CAD build for the part. Positions are in the model's coordinates, mm. Face numbers are marked on the shaded views. Round coordinates to 2 decimals unless told otherwise and drop trailing zeros. Write each loop counter-clockwise with the first axis right and the second up, starting at its lowest first coordinate (ties: lowest second). Pieces come first, ordered by that corner, then holes. Notation, with made-up numbers: (38.5, 12.25) - (72.5, 12.25) arc R26 ccw to (72.5, 35.25) - close; hole circle Ø4 at (-10.5, 45). An arc over 180 degrees is marked (long way). Put each result on its own line as item: value. Start each with the question number.
Item 1: Cut at B-B (y = 20). Give the cut face in (x, z).
Item 2: Drill centre lines: line 1 (Y direction, x = -27.5, z = 2.75); line 2 (X direction, y = -9, z = 1.65); line 3 (Y direction, x = -4, z = 1.15). Where is each one in solid material? Low to high. Write a range as from..to.
Item 3: Cut at C-C (x = -50.5). Give the cut face in (y, z), and give its area (3 significant figures).
Item 4: Cut at A-A (z = 1.55). Count the separate pieces of the cut face and the enclosed holes in it, and give its area (3 significant figures).
Item 5: Pin check, flat tip, straight feed: pin 1 Ø1.5 at (y, z) = (10.5, 1.5) entering from +X. Stop position of the tip, or through.
Item 6: Mould opens along Z. For the marked faces 1 and 2 say: released by +Z, released by -Z, zero draft, split by the parting line, or undercut.
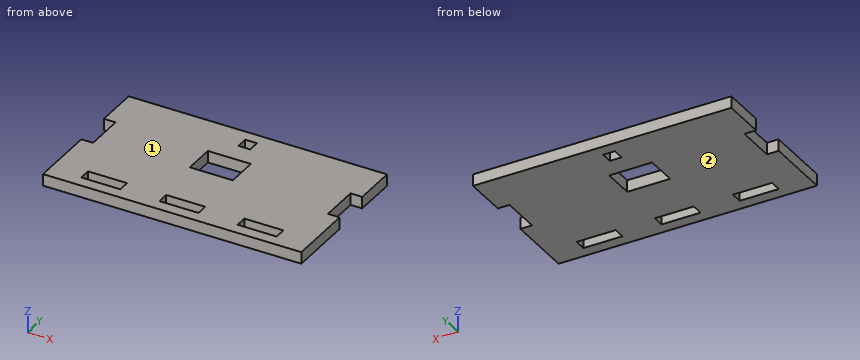
```python
from build123d import *

# Parameters (mm, degrees)
SKETCH1_W           = 10
SKETCH1_H           = 3
SKETCH1_W_2         = 11
SKETCH1_H_2         = 8
SKETCH1_W_3         = 3
BOSS_EXTRUDE1_DEPTH = 3


with BuildPart() as part:
    # Sketch1 → Boss-Extrude1 (new body)
    with BuildSketch(Plane.XY):
        Polygon((4.993890114, 24.809336695), (-61.106109886, 24.809336695), (-61.106109886, 13.809336695), (-58.106109886, 13.809336695), (-58.106109886, 3.809336695), (-61.106109886, 3.809336695), (-61.106109886, -13.190663305), (4.993890114, -13.190663305), (4.993890114, 3.809336695), (1.993890114, 3.809336695), (1.993890114, 13.809336695), (4.993890114, 13.809336695), align=None)
        with Locations((-28.056109886, -8.690663305)):
            Rectangle(SKETCH1_W, SKETCH1_H, mode=Mode.SUBTRACT)
        with Locations((-28.856109886, 9.559336695)):
            Rectangle(SKETCH1_W_2, SKETCH1_H_2, mode=Mode.SUBTRACT)
        with Locations((-28.056109886, 20.309336695)):
            Rectangle(SKETCH1_W_3, SKETCH1_H, mode=Mode.SUBTRACT)
        with Locations((-8.056109886, -8.690663305)):
            Rectangle(SKETCH1_W, SKETCH1_H, mode=Mode.SUBTRACT)
        with Locations((-48.056109886, -8.690663305)):
            Rectangle(SKETCH1_W, SKETCH1_H, mode=Mode.SUBTRACT)
    extrude(amount=BOSS_EXTRUDE1_DEPTH)


solid = part.part
```
Output values:
1. outline: (-61.11, 0) - (-29.56, 0) - (-29.56, 3) - (-61.11, 3) - close; (-26.56, 0) - (4.99, 0) - (4.99, 3) - (-26.56, 3) - close
2. line 1: -13.19..-10.19, -7.19..5.56, 13.56..18.81, 21.81..24.81
2. line 2: -61.11..-53.06, -43.06..-33.06, -23.06..-13.06, -3.06..4.99
2. line 3: -13.19..-10.19, -7.19..24.81
3. outline: (-13.19, 0) - (-10.19, 0) - (-10.19, 3) - (-13.19, 3) - close; (-7.19, 0) - (24.81, 0) - (24.81, 3) - (-7.19, 3) - close
3. area: 105 mm2
4. separate pieces: 1
4. enclosed holes: 5
4. area: 2,260 mm2
5. pin 1: x = 1.99
6. face 1: released by +Z
6. face 2: released by -Z
